Verification items for the finished model (mm, model axes). Face numbers are marked on the shaded views. A direction names the side the tool comes from. Give positions to 0.01 mm unless a question says otherwise; leave off trailing zeros. Order: outer loops, then holes, each group sorted by start corner. A loop starts at its lowest first (then second) coordinate and runs counter-clockwise, first axis right, second up. Notation, with made-up numbers: (81, -39) - (135, -39) arc R26 ccw to (135, -11) - close; hole circle Ø3 at (14.25, 77.5). An arc over 180 degrees is marked (long way). Answer as a JSON object with one key per item and string values.
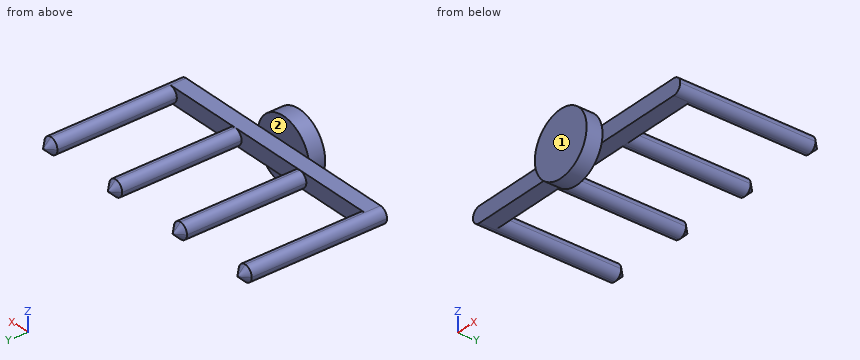
```python
from build123d import *

# Parameters (mm, degrees)
F0_W     = 6.35
F0_H     = 3.175
F0_W_2   = 3.175
F0_H_2   = 25.4
F2_DEPTH = 1.5875
F3_R     = 1.58749
F4_SIZE  = 1.58749


# Not quite as in the source:
# - a fillet or chamfer is up to 0.001 mm smaller than in the source, because OpenCascade refuses the exact size


with BuildPart() as f1:
    # F0 (on Top) → F1 (revolve)
    with BuildSketch(Plane.XY):
        with Locations((-11.7053389192, 22.0213071685)):
            Rectangle(F0_W, F0_H)
    revolve(axis=Axis((-8.5303389192, 22.0213071685, 0), (0, -1, 0)))

    # F0 (on Top) → F2 (join, symmetric)
    with BuildSketch(Plane.XY):
        Polygon((-33.9303389192, 23.6088071685), (-14.8803389192, 23.6088071685), (-8.5303389192, 23.6088071685), (-2.1803389192, 23.6088071685), (16.8696610808, 23.6088071685), (16.8696610808, 26.7838071685), (13.6946610808, 26.7838071685), (0.9946610808, 26.7838071685), (-2.1803389192, 26.7838071685), (-8.5303389192, 26.7838071685), (-14.8803389192, 26.7838071685), (-18.0553389192, 26.7838071685), (-30.7553389192, 26.7838071685), (-33.9303389192, 26.7838071685), align=None)
        with Locations((-32.3428389192, 39.4838071685)):
            Rectangle(F0_W_2, F0_H_2)
        with Locations((-16.4678389192, 39.4838071685)):
            Rectangle(F0_W_2, F0_H_2)
        with Locations((-0.5928389192, 39.4838071685)):
            Rectangle(F0_W_2, F0_H_2)
        with Locations((15.2821610808, 39.4838071685)):
            Rectangle(F0_W_2, F0_H_2)
    extrude(amount=F2_DEPTH, both=True)

    # F3 (radius 1.5875 in the source; OpenCascade refuses exactly that, so slightly less here)
    f3_edges = [f1.edges().sort_by_distance(p)[0] for p in [
        (-33.930339, 37.896307, 1.5875),
        (-33.930339, 37.896307, -1.5875),
        (-30.755339, 39.483807, 1.5875),
        (-30.755339, 39.483807, -1.5875),
        (-18.055339, 39.483807, 1.5875),
        (-18.055339, 39.483807, -1.5875),
        (-14.880339, 39.483807, 1.5875),
        (-14.880339, 39.483807, -1.5875),
        (-2.180339, 39.483807, 1.5875),
        (-2.180339, 39.483807, -1.5875),
        (0.994661, 39.483807, -1.5875),
        (0.994661, 39.483807, 1.5875),
        (16.869661, 37.896307, -1.5875),
        (16.869661, 37.896307, 1.5875),
        (13.694661, 39.483807, 1.5875),
        (13.694661, 39.483807, -1.5875),
    ]]
    fillet(f3_edges, radius=F3_R)

    # F4 (size 1.5875 in the source; OpenCascade refuses exactly that, so slightly less here)
    f4_edges = [f1.edges().sort_by_distance(p)[0] for p in [
        (-33.465374, 52.183807, -1.122535),
        (-17.590374, 52.183807, -1.122535),
        (-1.715374, 52.183807, -1.122535),
        (16.404696, 52.183807, -1.122535),
    ]]
    chamfer(f4_edges, length=F4_SIZE)


solid = f1.part
```
(1) Access from +Z, -Z, +X, -X, +Y, -Y to the whole of each face (thin tool, end or side, straight path). Record for the marked faces 1 and 2.
Computed values:
{"face 1": "+Z, -Z, +X, -X, -Y", "face 2": "+Z, +X, -X, +Y"}
(2) Section check C-C (z = -5.25). Record the cut outline in (x, y).
Computed values:
{"outline": "(-12.1, 20.43) - (-4.96, 20.43) - (-4.96, 23.61) - (-12.1, 23.61) - close"}
(3) Material ranges on line 1 along Y through (x, z) = (5, 1.25); line 2 along X through (y, z) = (34.5, -0.25); line 3 along Y through (x, z) = (-13.5, 3), recorded low to high. Write a range as [from, to].
Computed values:
{"line 1": "y = [23.61, 26.78]", "line 2": "x = [-33.91, -30.78], [-18.04, -14.9], [-2.16, 0.97], [13.71, 16.85]", "line 3": "y = [20.43, 23.61]"}
(4) Gauge pin test, flat ends, axial feed: pin 1 Ø2 at (x, z) = (-3, 2.5) entering from +Y; pin 2 Ø3 at (y, z) = (35.5, 2) entering from +X; pin 3 Ø6 at (x, y) = (1.5, 27.5) entering from -Z; pin 4 Ø1 at (y, z) = (35, -0.5) entering from -X. Record the tip position at first contact, or that the pin passes through.
Computed values:
{"pin 1": "stops at y = 26.78", "pin 2": "stops at x = 16.79", "pin 3": "stops at z = -1.59", "pin 4": "stops at x = -33.93"}
(5) Section check A-A (y = 37.5). Count the separate pieces of the cut face and the enclosed holes in it, then the cut area to 3 significant figures.
Computed values:
{"separate pieces": "4", "enclosed holes": "0", "area": "31.7 mm²"}
(6) Section check B-B (x = -8). Record the cut outline in (y, z).
Computed values:
{"outline": "(20.43, -6.33) - (23.61, -6.33) - (23.61, -1.59) - (26.78, -1.59) - (26.78, 1.59) - (23.61, 1.59) - (23.61, 6.33) - (20.43, 6.33) - close"}
(7) Section check D-D (x = -20). Record the cut outline in (y, z).
Computed values:
{"outline": "(23.61, -1.59) - (26.78, -1.59) - (26.78, 1.59) - (23.61, 1.59) - close"}
